Autodesk Inventor part; units mm, degrees
ref_plane "YZ Plane" through (0, 0, 0) normal (1, 0, 0) x (0, 1, 0)
ref_plane "XZ Plane" through (0, 0, 0) normal (0, 1, 0) x (-1, 0, 0)
ref_plane "XY Plane" through (0, 0, 0) normal (0, 0, 1) x (1, 0, 0)
sketch "Sketch1" plane through (0, 0, 0) normal (0, 1, 0) x (-1, 0, 0)
  line L0 (22.5, 5) -> (-22.5, 5)
  line L1 (-22.5, 5) -> (-22.5, -5)
  line L2 (-22.5, -5) -> (22.5, -5)
  line L3 (22.5, -5) -> (22.5, 5)
  line L4 (22.5, 5) -> (17.5, 5) construction
  line L5 (17.5, 5) -> (17.5, 0) construction
  circle A0 centre (17.5, 0) radius 1.6
  line L6 (0, -5) -> (0, -10.3319) construction
  circle A1 centre (-17.5, 0) radius 1.6
  point P0 (0, 0)
  dimension "d2" = 5
  dimension "d3" = 3.2
extrude "Extrusion1" add sketch "Sketch1" along normal blind 2.5
fillet "Fillet1" radius 1.5 4 edges at (-22.5, 1.25, 5) (22.5, 1.25, 5) (22.5, 1.25, -5) (-22.5, 1.25, -5)
sketch "Sketch5" plane through (0, 2.5, 0) normal (0, 1, 0) x (1, 0, 0)
  line L0 (0, 0) -> (-1, 0) construction
  line L1 (0, 0) -> (1, 0) construction
  line L2 (-1, 5) -> (-3, 5)
  line L3 (-3, 5) -> (-3, -5)
  line L4 (-21, -5) -> (21, -5)
  line L5 (-3, -5) -> (-1, -5)
  line L6 (-1, -5) -> (-1, 5)
  line L7 (21, 5) -> (-21, 5)
  line L8 (0, 0) -> (0, 0.5432) construction
  line L9 (1, 5) -> (3, 5)
  line L10 (3, 5) -> (3, -5)
  line L11 (21, -5) -> (-21, -5)
  line L12 (3, -5) -> (1, -5)
  line L13 (1, -5) -> (1, 5)
  dimension "d33" = 2
extrude "Extrusion5" add sketch "Sketch5" along normal blind 5 contours L6 L4 L3 L2 | L7 L10 L4 L13
sketch "Sketch6" plane through (3, 2.5, 5) normal (1, 0, 0) x (0, 0, -1)
  line L0 (10, -2.5) -> (10, 0) construction
  line L1 (-0.0046, 4.9481) -> (10, 0) construction
  line L2 (10, 5) -> (0, 5) construction
  line L3 (10, 5) -> (0, 0) construction
  line L4 (4.9728, 2.4864) -> (4.9728, 3.4864) construction
  line L5 (4.9728, 2.4864) -> (2.4728, 2.4864) construction
  circle A0 centre (2.4728, 2.4864) radius 1.1
  circle A1 centre (7.4728, 2.4864) radius 1.1
  line L6 (0, 5) -> (10, 5)
  line L7 (10, 5) -> (10, 0)
  line L8 (10, 0) -> (0, 0)
  line L9 (0, 0) -> (0, 5)
  point P0 (5, -2.5)
  dimension "d38" = 2.2
extrude "Extrusion6" cut sketch "Sketch6" against normal blind 6 contours A0 | A1
fillet "Fillet6" radius 1 4 edges at (-2, 7.5, 5) (2, 7.5, 5) (2, 7.5, -5) (-2, 7.5, -5)
fillet "Fillet7" radius 0.5 4 edges at (-3, 2.5, 0) (-1, 2.5, 0) (3, 2.5, 0) (1, 2.5, 0)
properties part number "CarbonConnectorPlateConnector"
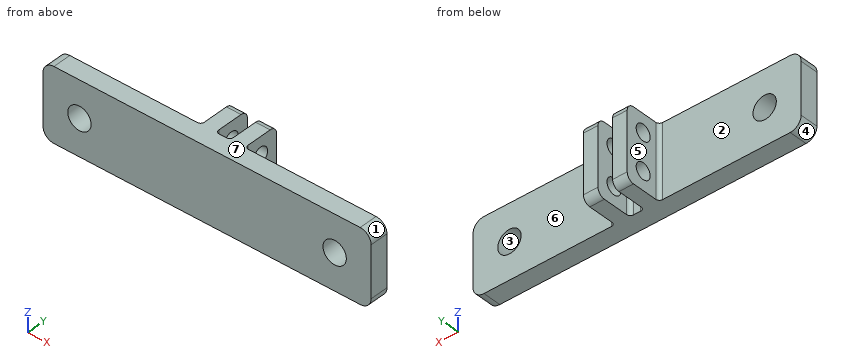
Input: part model. Units: mm. Frame: model coordinates. Face numbers are marked on the shaded views. A direction names the side the tool comes from. Coordinates: 2 decimals unless noted, no trailing zeros. Loops run counter-clockwise (first coordinate to the right, second up) from the corner with the lowest first, then second, coordinate; pieces in that order, holes last.
(1) Set-up query: the marked faces 5, 6 and 7. Return all of +Z, -Z, +X, -X, +Y, -Y with unobstructed straight access to the full face (end or side cutting, diameter ignored); none if empty.
(2) Section D-D on y = 5.5. Return the cut outline in (x, z).
(3) Section A-A on z = 0. Return the cut outline in (x, y), then the cut area to 3 significant figures.
(4) Material intervals for probe 1 along Z at (x, y) = (-17.5, 1.5); probe 2 along X at (y, z) = (1.75, -0.75); probe 3 along Y at (x, z) = (-18, 4.5), sorted ascending.
(5) Section B-B on x = -17.5. Return the cut outline in (y, z), then the cut area to 3 significant figures.
(6) Section C-C on y = 1.5. Return the cut outline in (x, z), then the cut area to 3 significant figures.
(7) First-contact query: pin 1 Ø2.5 at (x, z) = (17.5, 0) entering from -Y; pin 2 Ø2 at (y, z) = (5, 1) entering from +X; pin 3 Ø1.3 at (y, z) = (6, 1) entering from -X; pin 4 Ø3 at (x, z) = (14.5, 1) entering from +Y. Flat tips, straight axial feed; report the tip coordinate or a pass-through.
(8) Pull-direction query (X, two-part tool) for the marked faces 1, 2, 3 and 4; classes: released by +X, released by -X, zero draft, split by the parting line, or undercut.
Data:
1. face 5: +Z, -Z, -X, +Y
1. face 6: +Z, -Z, +X, +Y
1. face 7: +Z, +X, -X, +Y, -Y
2. outline: (-3, -5) - (-1, -5) - (-1, -3.45) - (-3, -3.45) - close; (-3, -1.5) - (-1, -1.5) - (-1, 1.55) - (-3, 1.55) - close; (-3, 3.5) - (-1, 3.5) - (-1, 5) - (-3, 5) - close; (1, -5) - (3, -5) - (3, -3.45) - (1, -3.45) - close; (1, -1.5) - (3, -1.5) - (3, 1.55) - (1, 1.55) - close; (1, 3.5) - (3, 3.5) - (3, 5) - (1, 5) - close
3. outline: (-22.5, 0) - (-19.1, 0) - (-19.1, 2.5) - (-22.5, 2.5) - close; (-15.9, 0) - (15.9, 0) - (15.9, 2.5) - (3.5, 2.5) arc R0.5 cw to (3, 3) - (3, 7.5) - (1, 7.5) - (1, 3) arc R0.5 cw to (0.5, 2.5) - (-0.5, 2.5) arc R0.5 cw to (-1, 3) - (-1, 7.5) - (-3, 7.5) - (-3, 3) arc R0.5 cw to (-3.5, 2.5) - (-15.9, 2.5) - close; (19.1, 0) - (22.5, 0) - (22.5, 2.5) - (19.1, 2.5) - close
3. area: 117 mm2
4. probe 1: z = -5 to -1.6, 1.6 to 5
4. probe 2: x = -22.5 to -18.91, -16.09 to 16.09, 18.91 to 22.5
4. probe 3: y = 0 to 2.5
5. outline: (0, -5) - (2.5, -5) - (2.5, -1.6) - (0, -1.6) - close; (0, 1.6) - (2.5, 1.6) - (2.5, 5) - (0, 5) - close
5. area: 17.0 mm2
6. outline: (-22.5, -3.5) arc R1.5 ccw to (-21, -5) - (21, -5) arc R1.5 ccw to (22.5, -3.5) - (22.5, 3.5) arc R1.5 ccw to (21, 5) - (-21, 5) arc R1.5 ccw to (-22.5, 3.5) - close; hole circle Ø3.2 at (-17.5, 0); hole circle Ø3.2 at (17.5, 0)
6. area: 432 mm2
7. pin 1: passes through
7. pin 2: stops at x = 3
7. pin 3: stops at x = -3
7. pin 4: stops at y = 2.5
8. face 1: released by +X
8. face 2: zero draft
8. face 3: undercut
8. face 4: released by -X
